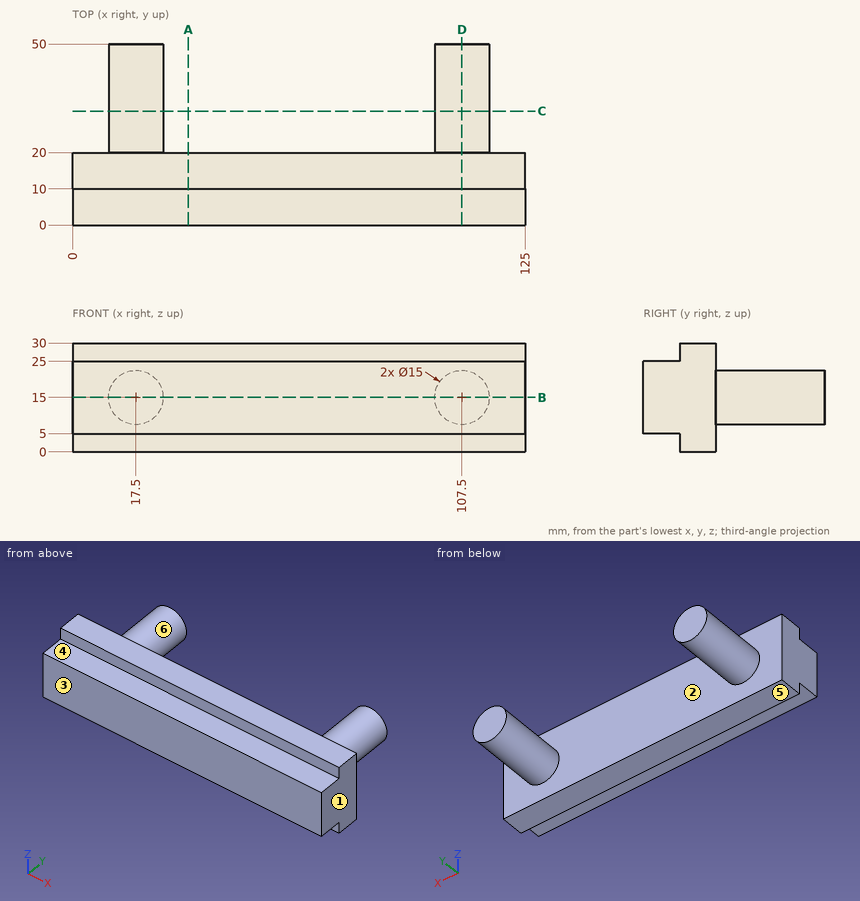
Source: three-view drawing plus pictorial views. Frame: mm from the lowest corner of the part. A direction names the side the tool comes from. Coordinates: 2 decimals unless noted, no trailing zeros. Loops run counter-clockwise (first coordinate to the right, second up) from the corner with the lowest first, then second, coordinate; pieces in that order, holes last. Notation, with made-up numbers: (-28.5, 72) - (-7.5, 72) arc R17 cw to (-7.5, 81) - close; hole circle Ø1 at (-12.5, 38). An arc over 180 degrees is marked (long way). One line per item, written item: value. Start each with the question number.
1. Section B-B (z = 15). Return the cut outline in (x, y), and give its area (3 significant figures).
2. Contact query for flat-ended pins moving along their axis: P1, Ø3, axis at y = 39.5, z = 10, coming from the -X side; P2, Ø5, axis at x = 46.5, z = 9, coming from the +Y side; P3, Ø3, axis at y = 44.5, z = 21.5, coming from the +X side; P4, Ø2, axis at x = 98, z = 21, coming from the -Y side. Output: stop coordinate, or through.
3. Set-up query: the marked faces 4, 5 and 6. Return all of +Z, -Z, +X, -X, +Y, -Y with unobstructed straight access to the full face (end or side cutting, diameter ignored); none if empty.
4. Section C-C (y = 31.5). Return the cut outline in (x, z), and give its area (3 significant figures).
5. Mould query, pull axis X, two halves, no side actions, for the marked faces 1, 2 and 3. Classes: pulls with the +X half, pulls with the -X half, needs draft (parallel to the pull), parting line crosses it, or undercut.
6. Section D-D (x = 107.5). Return the cut outline in (y, z).
7. Ray query, L1, parallel to Y at x = 7, z = 3.5; L2, parallel to X at y = 36, z = 12; L3, parallel to X at y = 44, z = 17. Return the intervals inside material, ascending.
8. Section A-A (x = 32). Return the cut outline in (y, z).
Verdict:
1. outline: (0, 0) - (125, 0) - (125, 20) - (115, 20) - (115, 50) - (100, 50) - (100, 20) - (25, 20) - (25, 50) - (10, 50) - (10, 20) - (0, 20) - close
1. area: 3,400 mm2
2. P1: stops at x = 10.87
2. P2: stops at y = 20
2. P3: stops at x = 113.09
2. P4: stops at y = 0
3. face 4: +Z, +X, -X, -Y
3. face 5: -Z, +X, -X, +Y, -Y
3. face 6: +Y
4. outline: circle Ø15 at (17.5, 15); circle Ø15 at (107.5, 15)
4. area: 353 mm2
5. face 1: pulls with the +X half
5. face 2: undercut
5. face 3: needs draft
6. outline: (0, 5) - (10, 5) - (10, 0) - (20, 0) - (20, 7.5) - (50, 7.5) - (50, 22.5) - (20, 22.5) - (20, 30) - (10, 30) - (10, 25) - (0, 25) - close
7. L1: y = 10 to 20
7. L2: x = 10.63 to 24.37, 100.63 to 114.37
7. L3: x = 10.27 to 24.73, 100.27 to 114.73
8. outline: (0, 5) - (10, 5) - (10, 0) - (20, 0) - (20, 30) - (10, 30) - (10, 25) - (0, 25) - close
